```python
from build123d import *

# Parameters (mm, degrees)
F0_R     = 4.6841242686
F1_DEPTH = 4.9
F2_R     = 7.8548268631
F3_DEPTH = 1.7
F4_T     = 2.5


# Not quite as in the source:
# - a shell that OpenCascade refuses in one call is made with other operations: the cavity is built on its own and cut out


with BuildPart() as f1:
    # F0 (on Top) → F1 (new body)
    with BuildSketch(Plane.XY):
        Circle(F0_R)
    extrude(amount=F1_DEPTH)

    # F2 (on face) → F3 (join)
    with BuildSketch(Plane(origin=(0, 0, 0), x_dir=(1, 0, 0), z_dir=(0, 0, -1))):
        Circle(F2_R)
    extrude(amount=F3_DEPTH)

    # F4: shell of thickness 2.5, made by hand


with BuildPart() as f4_core1:
    # F4_t2: copy of F1
    add(f1.part)

    # the walls: a layer under each face that stays
    f4_faces = [f4_core1.faces().sort_by_distance(p)[0] for p in [
        (-7.8548268631, 0, -0.85),
        (0, 0, -1.7),
        (-4.6841242686, 0, 2.45),
    ]]
    thicken(f4_faces, amount=-F4_T, mode=Mode.SUBTRACT)


with BuildPart() as f1_1:
    add(f1.part)

    # what is left inside the walls is the cavity
    f4_cavity = [f4_core1.part.solids().sort_by_distance(p)[0] for p in [
        (-2.159124, 0, 3.533333),
    ]]
    add(f4_cavity, mode=Mode.SUBTRACT)


solid = f1_1.part
```
Part model, mm, in its own coordinate system. A direction names the side the tool comes from. Round coordinates to 2 decimals unless told otherwise and drop trailing zeros. Loops run counter-clockwise (first coordinate to the right, second up) from the corner with the lowest first, then second, coordinate; pieces in that order, holes last.
Item 1: Mould opens along X. For faces 1 (the face through (0, 0, 0.8)), 2 (the face through (-3.717, -2.85, 2.416)), 3 (the face through (0, 0, -1.7)) say: +X half, -X half, draft (parallel to the pull), parting line (faces both ways), or undercut.
Item 2: Drop flat-ended pins along their axis: P1, Ø2, axis at x = -2, z = 3.5, coming from the +Y side; P2, Ø4, axis at x = 0, y = 0, coming from the +Z side; P3, Ø1.5, axis at x = 6, z = 2, coming from the +Y side; P4, Ø2, axis at x = -3.5, z = 1.5, coming from the -Y side. Give the stop position or say it passes through.
Item 3: Cut at D-D, the plane z = -1. Give the cut face in (x, y).
Item 4: Drill centre lines: line 1 (Y direction, x = 0, z = 2.8); line 2 (Z direction, x = -5, y = 0.25); line 3 (X direction, y = 2, z = 3.25). Where is each one in solid material? Low to high.
Item 5: 3-axis set-ups, long thin cutter, end or side, ignore diameter. For faces 4 (the face through (0, 5, 0)), 5 (the face through (-2.15, -0.98, 4.9)): which of +Z, -Z, +X, -X, +Y, -Y reach the whole face in a straight line?
Item 6: Cut at C-C, the plane z = 1. Give the cut face in (x, y), then the cut area to 3 significant figures.
Item 7: Cut at A-A, the plane x = 0. Give the cut face in (y, z), then the cut area to 3 significant figures.
A:
1. face 1: undercut
1. face 2: parting line
1. face 3: draft
2. P1: stops at y = 4.58
2. P2: stops at z = 0.8
2. P3: passes through
2. P4: stops at y = -3.96
3. outline: circle Ø15.71 at (0, 0)
4. line 1: y = -4.68 to -2.18, 2.18 to 4.68
4. line 2: z = -1.7 to 0
4. line 3: x = -4.24 to -0.88, 0.88 to 4.24
5. face 4: +Z
5. face 5: +Z, +X, -X, +Y, -Y
6. outline: circle Ø9.37 at (0, 0); hole circle Ø4.37 at (0, 0)
6. area: 53.9 mm2
7. outline: (-7.85, -1.7) - (7.85, -1.7) - (7.85, 0) - (4.68, 0) - (4.68, 4.9) - (2.18, 4.9) - (2.18, 0.8) - (-2.18, 0.8) - (-2.18, 4.9) - (-4.68, 4.9) - (-4.68, 0) - (-7.85, 0) - close
7. area: 54.7 mm2
